from build123d import *

# Parameters (mm, degrees)
SKETCH_1_R      = 5
EXTRUDE_1_DEPTH = 4


with BuildPart() as part:
    # Эскиз1 → Бобышка-Вытянуть1 (new body)
    with BuildSketch(Plane.XY):
        with BuildLine():
            Line((8.526879851, 0), (12, 0))
            ThreePointArc((12, 0), (14.121320344, 0.878679656), (15, 3))
            Line((15, 3), (15, 90))
            Line((15, 90), (19, 90))
            ThreePointArc((19, 90), (20.154255418, 88.845744582), (19, 87.691489165))
            Line((19, 87.691489165), (19, 3))
            ThreePointArc((19, 3), (19.878679656, 0.878679656), (22, 0))
            Line((22, 0), (134.07411748, 0))
            ThreePointArc((134.07411748, 0), (165, -14), (195.92588252, 0))
            Line((195.92588252, 0), (304.07411748, 0))
            ThreePointArc((304.07411748, 0), (335, -14), (365.92588252, 0))
            Line((365.92588252, 0), (478, 0))
            ThreePointArc((478, 0), (480.121320344, 0.878679656), (481, 3))
            Line((481, 3), (481, 87.691489165))
            ThreePointArc((481, 87.691489165), (479.845744582, 88.845744582), (481, 90))
            Line((481, 90), (485, 90))
            Line((485, 90), (485, 3))
            ThreePointArc((485, 3), (485.878679656, 0.878679656), (488, 0))
            Line((488, 0), (491.473120149, 0))
            ThreePointArc((491.473120149, 0), (498.004324615, 2.427459592), (501.364682095, 8.531326355))
            ThreePointArc((501.364682095, 8.531326355), (504.376413281, 95.021242555), (488, 180))
            Line((488, 180), (481, 180))
            Line((481, 180), (471, 170))
            Line((471, 170), (454.102752641, 170))
            Line((454.102752641, 170), (444.102752641, 180))
            Line((444.102752641, 180), (425, 180))
            Line((425, 180), (420, 175))
            Line((420, 175), (416, 175))
            Line((416, 175), (416, 171.109370144))
            ThreePointArc((416, 171.109370144), (415, 169.411148659), (414, 171.109370144))
            Line((414, 171.109370144), (414, 175))
            Line((414, 175), (410, 175))
            Line((410, 175), (405, 180))
            Line((405, 180), (395, 180))
            Line((395, 180), (390, 175))
            Line((390, 175), (386, 175))
            Line((386, 175), (386, 171.109370144))
            ThreePointArc((386, 171.109370144), (385, 169.411148659), (384, 171.109370144))
            Line((384, 171.109370144), (384, 175))
            Line((384, 175), (380, 175))
            Line((380, 175), (375, 180))
            Line((375, 180), (365, 180))
            Line((365, 180), (360, 175))
            Line((360, 175), (356, 175))
            Line((356, 175), (356, 171.109370144))
            ThreePointArc((356, 171.109370144), (355, 169.411148659), (354, 171.109370144))
            Line((354, 171.109370144), (354, 175))
            Line((354, 175), (350, 175))
            Line((350, 175), (345, 180))
            Line((345, 180), (335, 180))
            Line((335, 180), (330, 175))
            Line((330, 175), (326, 175))
            Line((326, 175), (326, 171.109370144))
            ThreePointArc((326, 171.109370144), (325, 169.411148659), (324, 171.109370144))
            Line((324, 171.109370144), (324, 175))
            Line((324, 175), (320, 175))
            Line((320, 175), (315, 180))
            Line((315, 180), (305, 180))
            Line((305, 180), (300, 175))
            Line((300, 175), (296, 175))
            Line((296, 175), (296, 171.109370144))
            ThreePointArc((296, 171.109370144), (295, 169.411148659), (294, 171.109370144))
            Line((294, 171.109370144), (294, 175))
            Line((294, 175), (290, 175))
            Line((290, 175), (285, 180))
            Line((285, 180), (275, 180))
            Line((275, 180), (270, 175))
            Line((270, 175), (266, 175))
            Line((266, 175), (266, 171.109370144))
            ThreePointArc((266, 171.109370144), (265, 169.411148659), (264, 171.109370144))
            Line((264, 171.109370144), (264, 175))
            Line((264, 175), (260, 175))
            Line((260, 175), (255, 180))
            Line((255, 180), (245, 180))
            Line((245, 180), (240, 175))
            Line((240, 175), (236, 175))
            Line((236, 175), (236, 171.109370144))
            ThreePointArc((236, 171.109370144), (235, 169.411148659), (234, 171.109370144))
            Line((234, 171.109370144), (234, 175))
            Line((234, 175), (230, 175))
            Line((230, 175), (225, 180))
            Line((225, 180), (215, 180))
            Line((215, 180), (210, 175))
            Line((210, 175), (206, 175))
            Line((206, 175), (206, 171.109370144))
            ThreePointArc((206, 171.109370144), (205, 169.411148659), (204, 171.109370144))
            Line((204, 171.109370144), (204, 175))
            Line((204, 175), (200, 175))
            Line((200, 175), (195, 180))
            Line((195, 180), (185, 180))
            Line((185, 180), (180, 175))
            Line((180, 175), (176, 175))
            Line((176, 175), (176, 171.109370144))
            ThreePointArc((176, 171.109370144), (175, 169.411148659), (174, 171.109370144))
            Line((174, 171.109370144), (174, 175))
            Line((174, 175), (170, 175))
            Line((170, 175), (165, 180))
            Line((165, 180), (155, 180))
            Line((155, 180), (150, 175))
            Line((150, 175), (146, 175))
            Line((146, 175), (146, 171.109370144))
            ThreePointArc((146, 171.109370144), (145, 169.411148659), (144, 171.109370144))
            Line((144, 171.109370144), (144, 175))
            Line((144, 175), (140, 175))
            Line((140, 175), (135, 180))
            Line((135, 180), (125, 180))
            Line((125, 180), (120, 175))
            Line((120, 175), (116, 175))
            Line((116, 175), (116, 171.109370144))
            ThreePointArc((116, 171.109370144), (115, 169.411148659), (114, 171.109370144))
            Line((114, 171.109370144), (114, 175))
            Line((114, 175), (110, 175))
            Line((110, 175), (105, 180))
            Line((105, 180), (95, 180))
            Line((95, 180), (90, 175))
            Line((90, 175), (86, 175))
            Line((86, 175), (86, 171.109370144))
            ThreePointArc((86, 171.109370144), (85, 169.411148659), (84, 171.109370144))
            Line((84, 171.109370144), (84, 175))
            Line((84, 175), (80, 175))
            Line((80, 175), (75, 180))
            Line((75, 180), (55.897247359, 180))
            Line((55.897247359, 180), (45.897247359, 170))
            Line((45.897247359, 170), (29, 170))
            Line((29, 170), (19, 180))
            Line((19, 180), (12, 180))
            ThreePointArc((12, 180), (-4.376413281, 95.021242555), (-1.364682095, 8.531326355))
            ThreePointArc((-1.364682095, 8.531326355), (1.995675385, 2.427459592), (8.526879851, 0))
        make_face()
        with Locations((45.897247359, 70)):
            Circle(SKETCH_1_R, mode=Mode.SUBTRACT)
        with Locations((65.46620575, 45)):
            Circle(SKETCH_1_R, mode=Mode.SUBTRACT)
        with Locations((75, 70)):
            Circle(SKETCH_1_R, mode=Mode.SUBTRACT)
        with Locations((94.568958391, 45)):
            Circle(SKETCH_1_R, mode=Mode.SUBTRACT)
        with Locations((104.102752641, 70)):
            Circle(SKETCH_1_R, mode=Mode.SUBTRACT)
        with Locations((123.671711032, 45)):
            Circle(SKETCH_1_R, mode=Mode.SUBTRACT)
        with Locations((133.205505282, 70)):
            Circle(SKETCH_1_R, mode=Mode.SUBTRACT)
        with Locations((152.774463674, 45)):
            Circle(SKETCH_1_R, mode=Mode.SUBTRACT)
        with Locations((162.308257923, 70)):
            Circle(SKETCH_1_R, mode=Mode.SUBTRACT)
        with Locations((181.877216315, 45)):
            Circle(SKETCH_1_R, mode=Mode.SUBTRACT)
        with Locations((191.411010565, 70)):
            Circle(SKETCH_1_R, mode=Mode.SUBTRACT)
        with Locations((210.979968956, 45)):
            Circle(SKETCH_1_R, mode=Mode.SUBTRACT)
        with Locations((220.513763206, 70)):
            Circle(SKETCH_1_R, mode=Mode.SUBTRACT)
        with Locations((240.082721597, 45)):
            Circle(SKETCH_1_R, mode=Mode.SUBTRACT)
        with Locations((249.616515847, 70)):
            Circle(SKETCH_1_R, mode=Mode.SUBTRACT)
        with Locations((269.185474238, 45)):
            Circle(SKETCH_1_R, mode=Mode.SUBTRACT)
        with Locations((278.719268488, 70)):
            Circle(SKETCH_1_R, mode=Mode.SUBTRACT)
        with Locations((298.288226879, 45)):
            Circle(SKETCH_1_R, mode=Mode.SUBTRACT)
        with Locations((307.822021129, 70)):
            Circle(SKETCH_1_R, mode=Mode.SUBTRACT)
        with Locations((327.39097952, 45)):
            Circle(SKETCH_1_R, mode=Mode.SUBTRACT)
        with Locations((336.92477377, 70)):
            Circle(SKETCH_1_R, mode=Mode.SUBTRACT)
        with Locations((356.493732162, 45)):
            Circle(SKETCH_1_R, mode=Mode.SUBTRACT)
        with Locations((366.027526411, 70)):
            Circle(SKETCH_1_R, mode=Mode.SUBTRACT)
        with Locations((385.596484803, 45)):
            Circle(SKETCH_1_R, mode=Mode.SUBTRACT)
        with Locations((395.130279053, 70)):
            Circle(SKETCH_1_R, mode=Mode.SUBTRACT)
        with Locations((414.699237444, 45)):
            Circle(SKETCH_1_R, mode=Mode.SUBTRACT)
        with Locations((425, 70)):
            Circle(SKETCH_1_R, mode=Mode.SUBTRACT)
        with Locations((444.568958391, 45)):
            Circle(SKETCH_1_R, mode=Mode.SUBTRACT)
        with Locations((454.869720947, 70)):
            Circle(SKETCH_1_R, mode=Mode.SUBTRACT)
        with BuildLine():
            Line((152, 6), (178, 6))
            Line((178, 6), (178, 9))
            ThreePointArc((178, 9), (179.414213562, 12.414213562), (176, 11))
            Line((176, 11), (154, 11))
            ThreePointArc((154, 11), (150.585786438, 12.414213562), (152, 9))
            Line((152, 9), (152, 6))
        make_face(mode=Mode.SUBTRACT)
        with BuildLine():
            Line((322, 6), (348, 6))
            Line((348, 6), (348, 9))
            ThreePointArc((348, 9), (349.414213562, 12.414213562), (346, 11))
            Line((346, 11), (324, 11))
            ThreePointArc((324, 11), (320.585786438, 12.414213562), (322, 9))
            Line((322, 9), (322, 6))
        make_face(mode=Mode.SUBTRACT)
    extrude(amount=EXTRUDE_1_DEPTH)


solid = part.part
Build history of the part. All positions in model axes, mm. A direction names the side the tool comes from. Give positions to 0.01 mm unless a question says otherwise; leave off trailing zeros. Loops run counter-clockwise (first coordinate to the right, second up) from the corner with the lowest first, then second, coordinate; pieces in that order, holes last. Notation, with made-up numbers: (-23, 39.25) - (-3, 39.25) arc R22 ccw to (-3, 71.25) - close; hole circle Ø9 at (7.25, 29). An arc over 180 degrees is marked (long way). Write item = value, one per line. Start each with the question number.
1) Pull direction Y, two halves, no side cores. Call faces 1 (the cylindrical face through (1.921, 2.493, 1.972)), 2 (the cylindrical face through (302.827, 70.22, 1.972)), 3 (the flat face through (476, 175, 2)), 4 (the cylindrical face through (-4.28, 96.23, 1.97)): +Y half, -Y half, draft (parallel to the pull), parting line (faces both ways), or undercut.
2) Drop flat-ended pins along their axis: pin 1 Ø1.2 at (y, z) = (51, 1.5) entering from +X; pin 2 Ø6 at (x, y) = (269.19, 45) entering from +Z; pin 3 Ø1 at (x, z) = (155.5, 3) entering from -Y; pin 4 Ø1 at (x, z) = (237.5, 2) entering from -Y. Give the stop position or say it passes through.
3) Tool access for faces 5 (the flat face through (51, 175.1, 2)), 6 (the cylindrical face through (429.77, 71.5, 1.97)): list every direction of +Z, -Z, +X, -X, +Y, -Y with a clear straight run to the whole face (end or side of a thin tool).
4) Probe probe 1 along Y at (x, z) = (162.5, 0.25); probe 2 along Y at (x, z) = (425, 1.25); probe 3 along Y at (x, z) = (74, 2.7). List the from-to ranges inside material, lowest first. Write a range as from..to.
5) Band-saw the part on A-A on z = 1. Count the separate pieces of the cut face and the enclosed holes in it, plus the area to 3 significant figures.
6) Band-saw the part on B-B on y = 137.5. Give the cut face in (x, z), plus the area to 3 significant figures.
Final values:
q1.face_1 = -Y half
q1.face_2 = undercut
q1.face_3 = +Y half
q1.face_4 = parting line
q2.pin_1 = 505.3
q2.pin_2 = through
q2.pin_3 = -13
q2.pin_4 = 0
q3.face_5 = +Z, -Z, +Y
q3.face_6 = +Z, -Z
q4.probe_1 = -13.92..6, 11..65, 75..180
q4.probe_2 = 0..65, 75..180
q4.probe_3 = 0..65.1, 74.9..180
q5.separate_pieces = 1
q5.enclosed_holes = 31
q5.area = 86,700 mm²
q6.outline = (1.33, 0) - (498.67, 0) - (498.67, 4) - (1.33, 4) - close
q6.area = 1,990 mm²
